Input: part model. Units: mm. Frame: model coordinates. Round coordinates to 2 decimals unless told otherwise and drop trailing zeros. Loops run counter-clockwise (first coordinate to the right, second up) from the corner with the lowest first, then second, coordinate; pieces in that order, holes last. Notation, with made-up numbers: M 77.25,38.5 L 101.25,38.5 A14 ccw 101.25,51.5 Z; hole C 49.5,-22 d4. An arc over 180 degrees is marked long. Use one line per item in the form item = value. Start each with the question number.
Q1. Ray query, line 1 along Y through (x, z) = (2.75, 63.5); line 2 along Z through (x, y) = (4.3, 0). Return the intervals inside material, ascending.
Q2. Section query B-B, the plane z = 15. Output: boundary loops of the cut face in (x, y), and give its area (3 significant figures).
Q3. Section query A-A, the plane y = 0. Output: boundary loops of the cut face in (x, z).
Q4. Section query C-C, the plane x = -3. Output: boundary loops of the cut face in (y, z), and give its area (3 significant figures).
Q5. First-contact query: P1, Ø4, axis at y = 0, z = 5, coming from the -X side. Flat tip, straight axial feed; report the tip coordinate or a pass-through.
Q6. Section query D-D, the plane z = 48.5. Output: boundary loops of the cut face in (x, y).
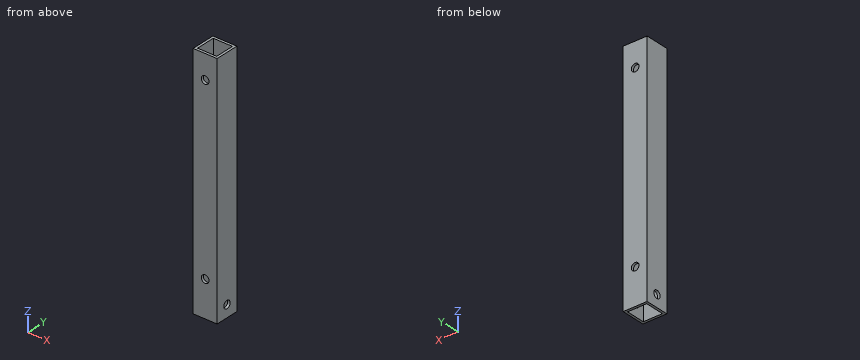
```python
from build123d import *

# Parameters (mm, degrees)
SKETCH_1_W          = 10
SKETCH_1_H          = 10
SKETCH_1_W_2        = 8
SKETCH_1_H_2        = 8
EXTRUDE_1_DEPTH     = 100
SKETCH_2_R          = 1.6
CUT_EXTRUDE_1_DEPTH = 101.623058987
SKETCH_3_R          = 1.6
CUT_EXTRUDE_2_DEPTH = 101.623058987
SKETCH_5_R          = 1.6
CUT_EXTRUDE_4_DEPTH = 101.623058987


with BuildPart() as part:
    # ｽｹｯﾁ1 → ﾎﾞｽ - 押し出し1 (new body)
    with BuildSketch(Plane.XY):
        Rectangle(SKETCH_1_W, SKETCH_1_H)
        Rectangle(SKETCH_1_W_2, SKETCH_1_H_2, mode=Mode.SUBTRACT)
    extrude(amount=EXTRUDE_1_DEPTH)

    # ｽｹｯﾁ2 → ｶｯﾄ - 押し出し1 (cut, through all)
    with BuildSketch(Plane.ZY.offset(5)):
        with Locations(Location((5, 0, 0), (0, 0, 270))):
            Circle(SKETCH_2_R)
    extrude(amount=-CUT_EXTRUDE_1_DEPTH, mode=Mode.SUBTRACT)

    # ｽｹｯﾁ3 → ｶｯﾄ - 押し出し2 (cut, through all)
    with BuildSketch(Plane(origin=(0, 5, 0), x_dir=(1, 0, 0), z_dir=(0, 1, 0))):
        with Locations(Location((0, -90, 0), (0, 0, 270))):
            Circle(SKETCH_3_R)
    extrude(amount=-CUT_EXTRUDE_2_DEPTH, mode=Mode.SUBTRACT)

    # ｽｹｯﾁ5 → ｶｯﾄ - 押し出し4 (cut, through all)
    with BuildSketch(Plane(origin=(0, 5, 0), x_dir=(1, 0, 0), z_dir=(0, 1, 0))):
        with Locations(Location((0, -15, 0), (0, 0, 270))):
            Circle(SKETCH_5_R)
    extrude(amount=-CUT_EXTRUDE_4_DEPTH, mode=Mode.SUBTRACT)


solid = part.part
```
Results found:
q1.line_1 = -5 to -4, 4 to 5
q1.line_2 = 0 to 3.4, 6.6 to 100
q2.outline = M -5,-5 L -1.6,-5 L -1.6,-4 L -4,-4 L -4,4 L -1.6,4 L -1.6,5 L -5,5 Z; M 1.6,-5 L 5,-5 L 5,5 L 1.6,5 L 1.6,4 L 4,4 L 4,-4 L 1.6,-4 Z
q2.area = 29.6 mm²
q3.outline = M -5,0 L -4,0 L -4,3.4 L -5,3.4 Z; M -5,6.6 L -4,6.6 L -4,100 L -5,100 Z; M 4,0 L 5,0 L 5,3.4 L 4,3.4 Z; M 4,6.6 L 5,6.6 L 5,100 L 4,100 Z
q4.outline = M -5,0 L -4,0 L -4,100 L -5,100 Z; M 4,0 L 5,0 L 5,100 L 4,100 Z
q4.area = 200 mm²
q5.P1 = -5
q6.outline = M -5,-5 L 5,-5 L 5,5 L -5,5 Z; hole M -4,-4 L 4,-4 L 4,4 L -4,4 Z
